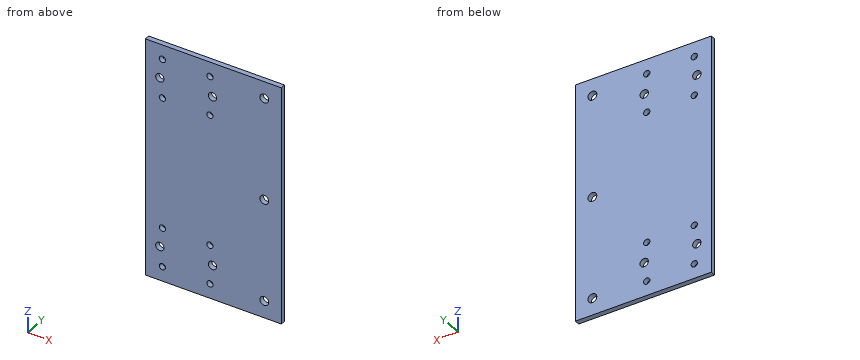
from build123d import *

# Parameters (mm, degrees)
SKETCH_1_R          = 2.5
SKETCH_1_R_2        = 2.45
SKETCH_1_R_3        = 1.85
SKETCH_1_W          = 48
SKETCH_1_H          = 40
EXTRUDE_1_DEPTH     = 3
SKETCH_2_R          = 2.6
CUT_EXTRUDE_1_DEPTH = 10


with BuildPart() as part:
    # 草图1 → 凸台-拉伸1 (new body)
    # profile 1 of 5: a face of its own
    with BuildSketch(Plane(origin=(0, 0, 0), x_dir=(1, 0, 0), z_dir=(0, 1, 0))):
        with BuildLine():
            Line((8, -30), (8, -70))
            Line((8, -70), (40, -70))
            Line((40, -70), (40, 60))
            Line((40, 60), (32.5, 60))
            ThreePointArc((32.5, 60), (28.232233047, 58.232233047), (30, 62.5))
            Line((30, 62.5), (30, 70))
            Line((30, 70), (8, 70))
            Line((8, 70), (8, 30))
            Line((8, 30), (-40, 30))
            Line((-40, 30), (-40, -30))
            Line((-40, -30), (8, -30))
        make_face()
        with Locations(Location((30, -60, 0), (0, 0, 270))):
            Circle(SKETCH_1_R, mode=Mode.SUBTRACT)
        with Locations(Location((30, 0, 0), (0, 0, 270))):
            Circle(SKETCH_1_R, mode=Mode.SUBTRACT)
    # profile 2 of 5: a face of its own
    with BuildSketch(Plane(origin=(0, 0, 0), x_dir=(1, 0, 0), z_dir=(0, 1, 0))):
        with BuildLine():
            Line((32.5, 60), (40, 60))
            Line((40, 60), (40, 70))
            Line((40, 70), (30, 70))
            Line((30, 70), (30, 62.5))
            ThreePointArc((30, 62.5), (31.767766953, 61.767766953), (32.5, 60))
        make_face()
    # profile 3 of 5: a face of its own
    with BuildSketch(Plane(origin=(0, 0, 0), x_dir=(1, 0, 0), z_dir=(0, 1, 0))):
        with BuildLine():
            Line((-40, 61.45), (-40, 30))
            Line((-40, 30), (8, 30))
            Line((8, 30), (8, 70))
            Line((8, 70), (-30, 70))
            Line((-30, 70), (-30, 63.3))
            ThreePointArc((-30, 63.3), (-28.691852455, 62.758147545), (-28.15, 61.45))
            ThreePointArc((-28.15, 61.45), (-30, 59.6), (-31.85, 61.45))
            Line((-31.85, 61.45), (-40, 61.45))
        make_face()
        with Locations(Location((-31.5, 50, 0), (0, 0, 270))):
            Circle(SKETCH_1_R_2, mode=Mode.SUBTRACT)
        with Locations(Location((-30, 38.55, 0), (0, 0, 270))):
            Circle(SKETCH_1_R_3, mode=Mode.SUBTRACT)
        with Locations(Location((-2, 38.55, 0), (0, 0, 270))):
            Circle(SKETCH_1_R_3, mode=Mode.SUBTRACT)
        with Locations(Location((-0.5, 50, 0), (0, 0, 270))):
            Circle(SKETCH_1_R_2, mode=Mode.SUBTRACT)
        with Locations(Location((-2, 61.45, 0), (0, 0, 270))):
            Circle(SKETCH_1_R_3, mode=Mode.SUBTRACT)
    # profile 4 of 5: a face of its own
    with BuildSketch(Plane(origin=(0, 0, 0), x_dir=(1, 0, 0), z_dir=(0, 1, 0))):
        with BuildLine():
            Line((-40, 70), (-40, 61.45))
            Line((-40, 61.45), (-31.85, 61.45))
            ThreePointArc((-31.85, 61.45), (-31.308147545, 62.758147545), (-30, 63.3))
            Line((-30, 63.3), (-30, 70))
            Line((-30, 70), (-40, 70))
        make_face()
    # profile 5 of 5: a face of its own
    with BuildSketch(Plane(origin=(0, 0, 0), x_dir=(1, 0, 0), z_dir=(0, 1, 0))):
        with Locations((-16, -50)):
            Rectangle(SKETCH_1_W, SKETCH_1_H)
        with Locations(Location((-30, -61.45, 0), (0, 0, 270))):
            Circle(SKETCH_1_R_3, mode=Mode.SUBTRACT)
        with Locations(Location((-31.5, -50, 0), (0, 0, 270))):
            Circle(SKETCH_1_R_2, mode=Mode.SUBTRACT)
        with Locations(Location((-30, -38.55, 0), (0, 0, 270))):
            Circle(SKETCH_1_R_3, mode=Mode.SUBTRACT)
        with Locations(Location((-2, -61.45, 0), (0, 0, 270))):
            Circle(SKETCH_1_R_3, mode=Mode.SUBTRACT)
        with Locations(Location((-0.5, -50, 0), (0, 0, 270))):
            Circle(SKETCH_1_R_2, mode=Mode.SUBTRACT)
        with Locations(Location((-2, -38.55, 0), (0, 0, 270))):
            Circle(SKETCH_1_R_3, mode=Mode.SUBTRACT)
    extrude(amount=EXTRUDE_1_DEPTH)

    # 草图2 → 切除-拉伸1 (cut)
    with BuildSketch(Plane(origin=(0, 3, 0), x_dir=(1, 0, 0), z_dir=(0, 1, 0))):
        with Locations(Location((30, 60, 0), (0, 0, 270))):
            Circle(SKETCH_2_R)
        with Locations(Location((30, 0, 0), (0, 0, 270))):
            Circle(SKETCH_2_R)
        with Locations(Location((30, -60, 0), (0, 0, 270))):
            Circle(SKETCH_2_R)
    extrude(amount=-CUT_EXTRUDE_1_DEPTH, mode=Mode.SUBTRACT)


solid = part.part
Geometry: final body of the model. Coordinates: model frame, mm. Round coordinates to 2 decimals unless told otherwise and drop trailing zeros. Loops run counter-clockwise (first coordinate to the right, second up) from the corner with the lowest first, then second, coordinate; pieces in that order, holes last. Notation, with made-up numbers: (62.5, 7) -> (77.5, 7) arc R32 cw to (77.5, 42) -> close; hole circle Ø10 at (40, 23). An arc over 180 degrees is marked (long way). One line per question, with ' | ' between items. Start each with the question number.
1. Section D-D on z = -38.55. Output: boundary loops of the cut face in (x, y), and give its area (3 significant figures).
2. Section C-C on y = 0.5. Count the separate pieces of the cut face and the enclosed holes in it, and give its area (3 significant figures).
3. Line query: line 1 along X through (y, z) = (1.8, 50); line 2 along X through (y, z) = (2, 38.55); line 3 along X through (y, z) = (0.95, 0). Output: solid intervals per line, ascending. Write a range as [from, to].
4. Contact query for a flat-ended pin moving along its axis: pin 1 (4.5 mm diameter, centred on x = -0.5, z = -50, fed in from -Y). Output: stop coordinate, or through.
5. Section B-B on x = 30. Output: boundary loops of the cut face in (y, z).
6. Section A-A on z = 50. Output: boundary loops of the cut face in (x, y).
Returned:
1) outline: (-40, 0) -> (-31.85, 0) -> (-31.85, 3) -> (-40, 3) -> close; (-28.15, 0) -> (-3.85, 0) -> (-3.85, 3) -> (-28.15, 3) -> close; (-0.15, 0) -> (40, 0) -> (40, 3) -> (-0.15, 3) -> close | area: 218 mm2
2) separate pieces: 1 | enclosed holes: 15 | area: 11,000 mm2
3) line 1: x = [-40, -33.95], [-29.05, -2.95], [1.95, 40] | line 2: x = [-40, -31.85], [-28.15, -3.85], [-0.15, 40] | line 3: x = [-40, 27.4], [32.6, 40]
4) pin 1: passes through
5) outline: (0, -70) -> (3, -70) -> (3, -62.6) -> (0, -62.6) -> close; (0, -57.4) -> (3, -57.4) -> (3, -2.6) -> (0, -2.6) -> close; (0, 2.6) -> (3, 2.6) -> (3, 57.4) -> (0, 57.4) -> close; (0, 62.6) -> (3, 62.6) -> (3, 70) -> (0, 70) -> close
6) outline: (-40, 0) -> (-33.95, 0) -> (-33.95, 3) -> (-40, 3) -> close; (-29.05, 0) -> (-2.95, 0) -> (-2.95, 3) -> (-29.05, 3) -> close; (1.95, 0) -> (40, 0) -> (40, 3) -> (1.95, 3) -> close
